Part model, mm, in its own coordinate system. Coordinates: 2 decimals unless noted, no trailing zeros. Loops run counter-clockwise (first coordinate to the right, second up) from the corner with the lowest first, then second, coordinate; pieces in that order, holes last. Notation, with made-up numbers: (0.5, 82.5) -> (41.5, 82.5) arc R18 ccw to (41.5, 92.5) -> close; hole circle Ø8 at (-11.75, 86). An arc over 180 degrees is marked (long way). Use one line per item in the form item = value. Start each with the question number.
(1) Band-saw the part on C-C on y = -10. Give the cut face in (x, z).
(2) Band-saw the part on B-B on x = -0.5. Give the cut face in (y, z).
(3) Pin check, flat tips, straight feed: P1, Ø14.5, axis at x = 23.42, y = -15.8, coming from the -Z side; P2, Ø12, axis at x = 13, y = -20, coming from the +Z side. Stop position of each tip, or through.
(4) Mould opens along Y. For faces 1 (the flat face through (-12, 3, 1)), 2 (the cylindrical face through (-12.11, 6.07, 0.49)) say: +Y half, -Y half, draft (parallel to the pull), parting line (faces both ways), or undercut.
(5) Drill centre lines: L1, parallel to Y at x = 0.5, z = 0.55; L2, parallel to X at y = -15.5, z = 0.6; L3, parallel to Y at x = -3, z = 0.2. Where is each one in solid material? Low to high. Write a range as [from, to].
(6) Band-saw the part on A-A on x = 32. Give the cut face in (y, z).
(7) Band-saw the part on D-D on z = 0.5. Give the cut face in (x, y).
```python
from build123d import *

# Parameters (mm, degrees)
F0_R     = 11
F1_DEPTH = 1
F2_R     = 12
F3_DEPTH = 25


with BuildPart() as f1:
    # F0 (on Top) → F1 (new body)
    with BuildSketch(Plane.XY):
        with BuildLine():
            ThreePointArc((-0.178199, 8.828474), (-7.956373, -9.949701), (10.821801, -2.171526))
            ThreePointArc((10.821801, -2.171526), (7.599976, 5.606648), (-0.178199, 8.828474))
        make_face()
        with BuildLine():
            ThreePointArc((-14.515293, -4.33895), (-36.118253, -22.921526), (-9.22379, -13.504102))
            ThreePointArc((-9.22379, -13.504102), (-0.002001, -16.670456), (9.140118, -13.280935))
            ThreePointArc((9.140118, -13.280935), (35.977676, -23.04613), (14.10199, -4.686721))
            ThreePointArc((14.10199, -4.686721), (11.937225, 5.795061), (3.171414, 11.936276))
            ThreePointArc((3.171414, 11.936276), (-0.178199, 40.544079), (-3.527811, 11.936276))
            ThreePointArc((-3.527811, 11.936276), (-12.195921, 5.941694), (-14.515293, -4.33895))
        make_face()
        with Locations((-23.560884, -15.671526)):
            Circle(F0_R, mode=Mode.SUBTRACT)
        with BuildLine():
            ThreePointArc((-0.178199, 8.828474), (7.599976, 5.606648), (10.821801, -2.171526))
            ThreePointArc((10.821801, -2.171526), (-7.956373, -9.949701), (-0.178199, 8.828474))
        make_face(mode=Mode.SUBTRACT)
        with Locations((23.420307, -15.79613)):
            Circle(F0_R, mode=Mode.SUBTRACT)
        with BuildLine():
            ThreePointArc((-0.178199, 15.044079), (-7.956373, 33.822254), (10.821801, 26.044079))
            ThreePointArc((10.821801, 26.044079), (7.599976, 18.265904), (-0.178199, 15.044079))
        make_face(mode=Mode.SUBTRACT)
    extrude(amount=F1_DEPTH)

    # F2 (on face) → F3 (cut)
    with BuildSketch(Plane.XY.offset(1)):
        with Locations((-0.178199, 26.044079)):
            Circle(F2_R)
        with Locations((-0.178199, -2.171526)):
            Circle(F2_R)
        with Locations((23.420307, -15.79613)):
            Circle(F2_R)
        with Locations((-23.560884, -15.671526)):
            Circle(F2_R)
    extrude(amount=-F3_DEPTH, mode=Mode.SUBTRACT)


solid = f1.part
```
A:
q1.outline = (-36.91, 0) -> (-34.14, 0) -> (-34.14, 1) -> (-36.91, 1) -> close; (-12.99, 0) -> (-9.27, 0) -> (-9.27, 1) -> (-12.99, 1) -> close; (8.92, 0) -> (12.91, 0) -> (12.91, 1) -> (8.92, 1) -> close; (33.93, 0) -> (36.71, 0) -> (36.71, 1) -> (33.93, 1) -> close
q2.outline = (-16.67, 0) -> (-14.17, 0) -> (-14.17, 1) -> (-16.67, 1) -> close; (9.82, 0) -> (14.05, 0) -> (14.05, 1) -> (9.82, 1) -> close; (38.04, 0) -> (40.54, 0) -> (40.54, 1) -> (38.04, 1) -> close
q3.P1 = through
q3.P2 = 1
q4.face_1 = draft
q4.face_2 = undercut
q5.L1 = [-16.66, -14.15], [9.81, 14.06], [38.02, 40.53]
q5.L2 = [-38.06, -35.56], [-11.56, -9.06], [-5.89, 5.53], [8.92, 11.42], [35.42, 37.92]
q5.L3 = [-16.39, -13.84], [9.49, 14.38], [37.71, 40.27]
q6.outline = (-27.49, 0) -> (-24.19, 0) -> (-24.19, 1) -> (-27.49, 1) -> close; (-7.41, 0) -> (-4.11, 0) -> (-4.11, 1) -> (-7.41, 1) -> close
q7.outline = (-14.52, -4.34) arc R14.5 ccw (long way) to (-9.22, -13.5) arc R14.5 ccw to (9.14, -13.28) arc R14.5 ccw (long way) to (14.1, -4.69) arc R14.5 ccw to (3.17, 11.94) arc R14.5 ccw (long way) to (-3.53, 11.94) arc R14.5 ccw to start; hole circle Ø24 at (-23.56, -15.67); hole circle Ø24 at (-0.18, -2.17); hole circle Ø24 at (-0.18, 26.04); hole circle Ø24 at (23.42, -15.8)
